Autodesk Fusion 360 part; units mm, degrees
sketch "Sketch1" plane through (0, 0, 0) normal (0, 1, 0) x (1, 0, 0) in component "Fast Light Board"
  line L0 (0, 0) -> (30.5594, 0)
  line L1 (30.5594, 0) -> (30.5594, 10.3188)
  line L2 (30.5594, 10.3188) -> (0, 10.3188)
  line L3 (0, 10.3188) -> (0, 0)
  circle A0 centre (4.7625, 5.1594) radius 1.9844
  dimension "d1" = 10.3188
  dimension "d2" = 30.5594
  dimension "d4" = 3.9688
extrude "Extrude1" add sketch "Sketch1" along normal blind 1.5875 in component "Fast Light Board"
sketch "Sketch2" plane through (0, 1.5875, 0) normal (0, 1, 0) x (-1, 0, 0) in component "Fast Light Board"
  circle A0 centre (-4.7625, -5.1594) radius 1.9844
  line L0 (0, -10.3188) -> (0, 0)
  line L1 (0, 0) -> (-30.5594, 0)
  line L2 (-30.5594, 0) -> (-30.5594, -10.3188)
  line L3 (-30.5594, -10.3188) -> (0, -10.3188)
  line L4 (-25.7969, -5.1594) -> (-25.7969, -7.5406)
  line L5 (-25.7969, -7.5406) -> (-30.5594, -7.5406)
  line L6 (-30.5594, -5.1594) -> (-30.5594, -7.5406)
  line L7 (-30.5594, -5.1594) -> (-30.5594, -2.7781)
  line L8 (-30.5594, -2.7781) -> (-25.7969, -2.7781)
  line L9 (-25.7969, -2.7781) -> (-25.7969, -5.1594)
  dimension "d7" = 4.7625
extrude "Extrude2" add sketch "Sketch2" along normal blind 1.5875 contours L2 L4 L5 L6 L7 L8 L9 in component "Fast Light Board"
sketch "Sketch3" plane through (0, 1.5875, 0) normal (0, 1, 0) x (-1, 0, 0) in component "Fast Light Board"
  line L0 (-25.7969, -7.5406) -> (-30.5594, -7.5406)
  line L1 (-30.5594, -7.5406) -> (-30.5594, -10.3188)
  line L2 (-30.5594, -10.3188) -> (0, -10.3188)
  line L3 (0, -10.3188) -> (0, 0)
  line L4 (0, 0) -> (-30.5594, 0)
  line L5 (-30.5594, 0) -> (-30.5594, -2.7781)
  line L6 (-30.5594, -2.7781) -> (-25.7969, -2.7781)
  line L7 (-25.7969, -2.7781) -> (-25.7969, -7.5406)
  circle A0 centre (-4.7625, -5.1594) radius 1.9844
  line L8 (-30.5594, -5.1594) -> (-17.8594, -5.1594)
  line L9 (-17.8594, -5.1594) -> (-19.1294, -5.1594)
  circle A1 centre (-19.1294, -5.1594) radius 0.5953
  circle A2 centre (-16.5894, -5.1594) radius 0.5953
  circle A3 centre (-19.1294, -7.6994) radius 0.5953
  circle A4 centre (-16.5894, -7.6994) radius 0.5953
  circle A5 centre (-16.5894, -2.6194) radius 0.5953
  circle A6 centre (-19.1294, -2.6194) radius 0.5953
  dimension "d12" = 12.7
  dimension "d13" = 1.27
  dimension "d14" = 1.1906
  dimension "d15" = 1.1906
  dimension "d16" = 1.1906
  dimension "d17" = 1.1906
  dimension "d18" = 1.1906
  dimension "d19" = 1.1906
extrude "Extrude3" cut sketch "Sketch3" against normal blind 1.5875 contours L8 L9 A1 | L8 L9 A1 | A2 | A3 | A4 | A5 | A6 in component "Fast Light Board"
component "Fast Light Board" placed x (1, 0, 0) y (0, 1, 0) z (0, 0, 1) at (0, 0, 0)
equation "d1 = ( 13 / 32 ) * 1 in"
equation "d2 = 1 13/64\""
equation "d4 = ( 5 / 32 ) * 1 in"
equation "d5 = ( 1 / 16 ) * 1 in"
equation "d7 = ( 3 / 16 ) * 1 in"
equation "d10 = ( 1 / 16 ) * 1 in"
equation "d14 = ( 3 / 64 ) * 1 in"
equation "d15 = ( 3 / 64 ) * 1 in"
equation "d16 = ( 3 / 64 ) * 1 in"
equation "d17 = ( 3 / 64 ) * 1 in"
equation "d18 = ( 3 / 64 ) * 1 in"
equation "d19 = ( 3 / 64 ) * 1 in"
equation "d20 = ( -1 / 16 ) * 1 in"
properties part number "fast-rgb-led-insert"
The listing builds one solid part. Answer for the finished solid, in the listing's coordinates (mm). A direction names the side the tool comes from. Round coordinates to 2 decimals unless told otherwise and drop trailing zeros. Loops run counter-clockwise (first coordinate to the right, second up) from the corner with the lowest first, then second, coordinate; pieces in that order, holes last.
Q1. Section B-B, the plane y = 1.2 is taken. Determine the outline of the cut face in (x, z), then the cut area to 3 significant figures.
Q2. Section D-D, the plane z = -0.5 is taken. Determine the outline of the cut face in (x, y).
Q3. Given pin 1 Ø1.7 at (x, y) = (27.5, 2.5) entering from +Z; pin 2 Ø1.5 at (x, z) = (16.59, -7.7) entering from +Y; pin 3 Ø1.3 at (x, y) = (28, 2.5) entering from -Z, each flat-ended and moving along its own axis, determine where each tip first touches the part or whether it passes through.
Q4. Section C-C, the plane x = 5 is taken. Determine the outline of the cut face in (y, z), then the cut area to 3 significant figures.
Q5. Section A-A, the plane x = 26.5 is taken. Determine the outline of the cut face in (y, z) (1 decimal).
Q6. Find the intervals of material crossed by line 1 (X direction, y = 1.55, z = -3); line 2 (X direction, y = 2.55, z = -3); line 3 (Y direction, x = 16.5, z = -4.5), in increasing order.
Q7. Which of the six approach directions +Z, -Z, +X, -X, +Y, -Y give full straight-line access (tool end or side, diameter ignored) to faces 1 (the face through (16.04, 0.8, -5.39)), 2 (the face through (28, 2, -2.778))?
Q8. For a pull along Z with two mould halves and no side action, classify faces 3 (the face through (25.797, 2, -5)), 4 (the face through (28, 2, -7.541)), 5 (the face through (5.68, 0.78, -6.92)), 6 (the face through (15, 1, 0)) as released by +Z, released by -Z, zero draft, split by the parting line, or undercut.
Completed:
1. outline: (0, -10.32) - (30.56, -10.32) - (30.56, 0) - (0, 0) - close; hole circle Ø3.97 at (4.76, -5.16); hole circle Ø1.19 at (16.59, -7.7); hole circle Ø1.19 at (16.59, -5.16); hole circle Ø1.19 at (16.59, -2.62); hole circle Ø1.19 at (19.13, -7.7); hole circle Ø1.19 at (19.13, -5.16); hole circle Ø1.19 at (19.13, -2.62)
1. area: 296 mm2
2. outline: (0, 0) - (30.56, 0) - (30.56, 1.59) - (0, 1.59) - close
3. pin 1: stops at z = -2.78
3. pin 2: stops at y = 1.59
3. pin 3: stops at z = -7.54
4. outline: (0, -10.32) - (1.59, -10.32) - (1.59, -7.13) - (0, -7.13) - close; (0, -3.19) - (1.59, -3.19) - (1.59, 0) - (0, 0) - close
4. area: 10.1 mm2
5. outline: (0, -10.3) - (1.6, -10.3) - (1.6, -7.5) - (3.2, -7.5) - (3.2, -2.8) - (1.6, -2.8) - (1.6, 0) - (0, 0) - close
6. line 1: x = 0 to 16.13, 17.05 to 18.67, 19.59 to 30.56
6. line 2: x = 25.8 to 30.56
6. line 3: y = 0 to 1.59
7. face 1: +Y, -Y
7. face 2: +Z, +X, -X, +Y
8. face 3: zero draft
8. face 4: released by -Z
8. face 5: undercut
8. face 6: released by +Z
